```python
from build123d import *

# Parameters (mm, degrees)
SKETCH_1_R          = 1.25
EXTRUDE_1_DEPTH     = 25
SKETCH_2_R          = 1.25
CUT_EXTRUDE_1_DEPTH = 25
SKETCH_3_R          = 1.25
CUT_EXTRUDE_2_DEPTH = 25


with BuildPart() as part:
    # Эскиз1 → Бобышка-Вытянуть1 (new body)
    with BuildSketch(Plane.XY):
        Polygon((0, 0), (0, 25), (25, 0), align=None)
        with Locations((5, 5)):
            Circle(SKETCH_1_R, mode=Mode.SUBTRACT)
    extrude(amount=EXTRUDE_1_DEPTH)

    # Эскиз2 → Вырез-Вытянуть1 (cut)
    with BuildSketch(Plane.ZY):
        with Locations((15, 10)):
            Circle(SKETCH_2_R)
    extrude(amount=-CUT_EXTRUDE_1_DEPTH, mode=Mode.SUBTRACT)

    # Эскиз3 → Вырез-Вытянуть2 (cut)
    with BuildSketch(Plane.XZ):
        with Locations((10, 10)):
            Circle(SKETCH_3_R)
    extrude(amount=-CUT_EXTRUDE_2_DEPTH, mode=Mode.SUBTRACT)


solid = part.part
```
Input: part model. Units: mm. Frame: model coordinates. Round coordinates to 2 decimals unless told otherwise and drop trailing zeros. Order: outer loops, then holes, each group sorted by start corner. A loop starts at its lowest first (then second) coordinate and runs counter-clockwise, first axis right, second up. Notation, with made-up numbers: (67, -19.5) - (106, -19.5) arc R18 ccw to (106, -2.5) - close; hole circle Ø8 at (-11, 26.5). An arc over 180 degrees is marked (long way). One line per question, with ' | ' between items. Start each with the question number.
1) Cut plane A-A, the plane y = 5. Return the cut outline in (x, z), then the cut area to 3 significant figures.
2) Pull-direction query (X, two-part tool) for faces 1 (the flat face through (7, 7, 0)), 2 (the cylindrical face through (8.75, 8.07, 10.05)), 3 (the flat face through (0, 12, 12)); classes: +X half, -X half, draft (parallel to the pull), parting line (faces both ways), or undercut.
3) Ray query, probe 1 along Z at (x, y) = (10, 12); probe 2 along Z at (x, y) = (8.5, 10); probe 3 along X at (y, z) = (4.5, 10). Return the intervals inside material, ascending.
4) Cut plane D-D, the plane x = 3. Return the cut outline in (y, z), then the cut area to 3 significant figures.
5) Cut plane C-C, the plane z = 10. Return the cut outline in (x, y).
6) Contact query for flat-ended pins moving along their axis: P1, Ø8, axis at x = 18.5, z = 5.5, coming from the -Y side; P2, Ø1, axis at y = 22.5, z = 5, coming from the +X side; P3, Ø3, axis at y = 14, z = 22.5, coming from the +X side; P4, Ø3, axis at y = 21.5, z = 13.5, coming from the +X side. Output: stop coordinate, or through.
7) Cut plane B-B, the plane x = 10. Return the cut outline in (y, z), then the cut area to 3 significant figures.
Worked out:
1) outline: (0, 0) - (3.75, 0) - (3.75, 25) - (0, 25) - close; (6.25, 0) - (20, 0) - (20, 25) - (6.25, 25) - close; hole circle Ø2.5 at (10, 10) | area: 433 mm^2
2) face 1: draft | face 2: undercut | face 3: -X half
3) probe 1: z = 0 to 8.75, 11.25 to 25 | probe 2: z = 0 to 13.75, 16.25 to 25 | probe 3: x = 0 to 3.85, 6.15 to 8.75, 11.25 to 20.5
4) outline: (0, 0) - (22, 0) - (22, 25) - (0, 25) - close; hole circle Ø2.5 at (10, 15) | area: 545 mm^2
5) outline: (0, 0) - (8.75, 0) - (8.75, 16.25) - (0, 25) - close; (11.25, 0) - (25, 0) - (11.25, 13.75) - close; hole circle Ø2.5 at (5, 5)
6) P1: stops at y = 0 | P2: stops at x = 3 | P3: stops at x = 12.5 | P4: stops at x = 5
7) outline: (0, 0) - (15, 0) - (15, 8.75) - (0, 8.75) - close; (0, 11.25) - (15, 11.25) - (15, 25) - (0, 25) - close; hole circle Ø2.5 at (10, 15) | area: 333 mm^2
